Part model, mm, in its own coordinate system. Face numbers are marked on the shaded views. A direction names the side the tool comes from. Round coordinates to 2 decimals unless told otherwise and drop trailing zeros. Loops run counter-clockwise (first coordinate to the right, second up) from the corner with the lowest first, then second, coordinate; pieces in that order, holes last. Notation, with made-up numbers: (-3.75, 22) - (19.25, 22) arc R33 cw to (19.25, 59) - close; hole circle Ø8 at (36.25, 9). An arc over 180 degrees is marked (long way). Put each result on its own line as item: value.
from build123d import *

# Parameters (mm, degrees)
CROQUIS1_W              = 35
CROQUIS1_H              = 35
SALIENTE_EXTRUIR2_DEPTH = 75.5
CROQUIS2_W              = 26.5
CROQUIS2_H              = 26.5
CORTAR_EXTRUIR1_DEPTH   = 80
CROQUIS4_R              = 1.25
CORTAR_EXTRUIR2_DEPTH   = 10
CORTAR_EXTRUIR5_START   = -10
CROQUIS9_R              = 1.25
CORTAR_EXTRUIR5_DEPTH   = 10
CROQUIS11_W             = 26.5
CROQUIS11_H             = 26.5
SALIENTE_EXTRUIR3_DEPTH = 37
CROQUIS13_W             = 26.5
CROQUIS13_H             = 26.5
CORTAR_EXTRUIR6_DEPTH   = 30
CORTAR_EXTRUIR7_REACH   = 47.768


with BuildPart() as part:
    # Croquis1 → Saliente-Extruir2 (new body)
    with BuildSketch(Plane.XY):
        Rectangle(CROQUIS1_W, CROQUIS1_H)
    extrude(amount=SALIENTE_EXTRUIR2_DEPTH)

    # Croquis2 → Cortar-Extruir1 (cut)
    with BuildSketch(Plane.XY.offset(75.5)):
        Rectangle(CROQUIS2_W, CROQUIS2_H)
    extrude(amount=-CORTAR_EXTRUIR1_DEPTH, mode=Mode.SUBTRACT)

    # Croquis4 → Cortar-Extruir2 (cut)
    with BuildSketch(Plane.XY.offset(75.5)):
        with Locations((-15.375, 15.38)):
            Circle(CROQUIS4_R)
        with Locations((15.38, 15.38)):
            Circle(CROQUIS4_R)
        with Locations((15.38, -15.38)):
            Circle(CROQUIS4_R)
        with Locations((-15.375, -15.38)):
            Circle(CROQUIS4_R)
    extrude(amount=-CORTAR_EXTRUIR2_DEPTH, mode=Mode.SUBTRACT)

    # Croquis9 → Cortar-Extruir5 (cut)
    with BuildSketch(Plane(origin=(0, 0, 0), x_dir=(-1, 0, 0), z_dir=(0, 0, -1)).offset(CORTAR_EXTRUIR5_START)):
        with Locations(Location((-15.38, 15.38, 0), (0, 0, 180))):
            Circle(CROQUIS9_R)
        with Locations((15.38, 15.38)):
            Circle(CROQUIS9_R)
        with Locations((15.38, -15.38)):
            Circle(CROQUIS9_R)
        with Locations(Location((-15.38, -15.38, 0), (0, 0, 180))):
            Circle(CROQUIS9_R)
    extrude(amount=CORTAR_EXTRUIR5_DEPTH, mode=Mode.SUBTRACT)

    # Croquis11 → Saliente-Extruir3 (add)
    with BuildSketch(Plane(origin=(0, 0, 0), x_dir=(-1, 0, 0), z_dir=(0, 0, -1))):
        Rectangle(CROQUIS11_W, CROQUIS11_H)
    extrude(amount=-SALIENTE_EXTRUIR3_DEPTH)

    # Croquis13 → Cortar-Extruir6 (cut)
    with BuildSketch(Plane(origin=(0, 0, 0), x_dir=(-1, 0, 0), z_dir=(0, 0, -1))):
        Rectangle(CROQUIS13_W, CROQUIS13_H)
    extrude(amount=-CORTAR_EXTRUIR6_DEPTH, mode=Mode.SUBTRACT)

    # Croquis14 → Cortar-Extruir7 (cut, up to next)
    with BuildSketch(Plane.XY.offset(37), mode=Mode.PRIVATE) as cortar_extruir7_sk1:
        with BuildLine():
            Line((13.25, -5.072292803), (13.25, 0))
            Line((13.25, 0), (-13.25, 0))
            Line((-13.25, 0), (-13.25, -5.072292803))
            Line((-13.25, -5.072292803), (-8.314710179, -8.652490661))
            ThreePointArc((-8.314710179, -8.652490661), (0, -11.350749828), (8.314710179, -8.652490661))
            Line((8.314710179, -8.652490661), (13.25, -5.072292803))
        make_face()
    cortar_extruir7_tool1 = extrude(cortar_extruir7_sk1.sketch, amount=-CORTAR_EXTRUIR7_REACH, mode=Mode.PRIVATE) & part.part
    # Croquis14 → Cortar-Extruir7 (cut, up to next)
    with BuildSketch(Plane.XY.offset(37), mode=Mode.PRIVATE) as cortar_extruir7_sk2:
        with BuildLine():
            Line((-13.25, 0), (13.25, 0))
            Line((13.25, 0), (13.25, 4.999749994))
            Line((13.25, 4.999749994), (8.314710179, 8.652490661))
            ThreePointArc((8.314710179, 8.652490661), (0, 11.394764723), (-8.314710179, 8.652490661))
            Line((-8.314710179, 8.652490661), (-13.25, 4.999749994))
            Line((-13.25, 4.999749994), (-13.25, 0))
        make_face()
    cortar_extruir7_tool2 = extrude(cortar_extruir7_sk2.sketch, amount=-CORTAR_EXTRUIR7_REACH, mode=Mode.PRIVATE) & part.part
    add(cortar_extruir7_tool1.solids().sort_by_distance((0, -4.780438, 37))[0], mode=Mode.SUBTRACT)
    add(cortar_extruir7_tool2.solids().sort_by_distance((0, 4.791209, 37))[0], mode=Mode.SUBTRACT)


solid = part.part
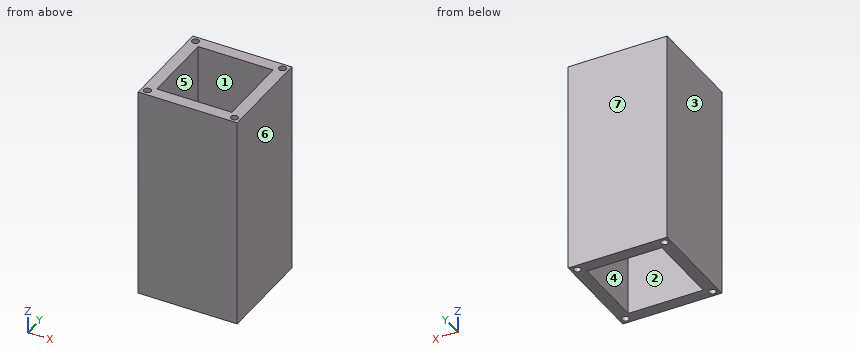
1. Two-plate mould, pull along X, no slides. Class the marked faces 4, 5, 6 and 7: pulls with the +X half, pulls with the -X half, needs draft (parallel to the pull), parting line crosses it, or undercut.
A:
face 4: undercut
face 5: undercut
face 6: pulls with the +X half
face 7: needs draft
2. Tool access for the marked faces 1, 2 and 3: list every direction of +Z, -Z, +X, -X, +Y, -Y with a clear straight run to the whole face (end or side of a thin tool).
A:
face 1: +Z
face 2: -Z
face 3: +Z, -Z, -X, +Y, -Y
3. Band-saw the part on B-B (z = 48.5). List the corners of the cut face in (x, y).
A:
outline: (-17.5, -17.5) - (17.5, -17.5) - (17.5, 17.5) - (-17.5, 17.5) - close; hole (-13.25, -13.25) - (13.25, -13.25) - (13.25, 13.25) - (-13.25, 13.25) - close
4. Band-saw the part on A-A (y = -3.5). List the corners of the cut face in (x, z).
A:
outline: (-17.5, 0) - (-13.25, 0) - (-13.25, 75.5) - (-17.5, 75.5) - close; (13.25, 0) - (17.5, 0) - (17.5, 75.5) - (13.25, 75.5) - close
5. Band-saw the part on D-D (z = 7.5). List the corners of the cut face in (x, y).
A:
outline: (-17.5, -17.5) - (17.5, -17.5) - (17.5, 17.5) - (-17.5, 17.5) - close; hole circle Ø2.5 at (-15.38, -15.38); hole circle Ø2.5 at (-15.38, 15.38); hole (-13.25, -13.25) - (13.25, -13.25) - (13.25, 13.25) - (-13.25, 13.25) - close; hole circle Ø2.5 at (15.38, -15.38); hole circle Ø2.5 at (15.38, 15.38)
6. Probe line 1 along Y through (x, z) = (-15.38, 3); line 2 along Y through (x, z) = (-7, 5.5). List the from-to ranges inside material, lowest first. Write a range as [from, to].
A:
line 1: y = [-17.5, -16.63], [-14.13, 14.13], [16.63, 17.5]
line 2: y = [-17.5, -13.25], [13.25, 17.5]
7. Pin check, flat tips, straight feed: P1, Ø6.5, axis at x = 6, y = 7, coming from the +Z side; P2, Ø0.8, axis at x = 15.5, y = 15.5, coming from the -Z side; P3, Ø2, axis at x = -15.375, y = -15.38, coming from the +Z side. Stop position of each tip, or through.
A:
P1: stops at z = 37
P2: stops at z = 10
P3: stops at z = 65.5
8. Band-saw the part on C-C (x = -10). List the corners of the cut face in (y, z).
A:
outline: (-17.5, 0) - (-13.25, 0) - (-13.25, 30) - (-7.43, 30) - (-7.43, 37) - (-13.25, 37) - (-13.25, 75.5) - (-17.5, 75.5) - close; (7.41, 30) - (13.25, 30) - (13.25, 0) - (17.5, 0) - (17.5, 75.5) - (13.25, 75.5) - (13.25, 37) - (7.41, 37) - close
